The listing builds one solid part. Answer for the finished solid, in the listing's coordinates (mm). Give positions to 0.01 mm unless a question says otherwise; leave off trailing zeros. Order: outer loops, then holes, each group sorted by start corner. A loop starts at its lowest first (then second) coordinate and runs counter-clockwise, first axis right, second up. Notation, with made-up numbers: (85.5, -25.5) - (118.5, -25.5) arc R22 cw to (118.5, -15.5) - close; hole circle Ø3 at (-9, 80.5). An arc over 180 degrees is marked (long way). Use CSV: the item, a comma, the result in double quotes.
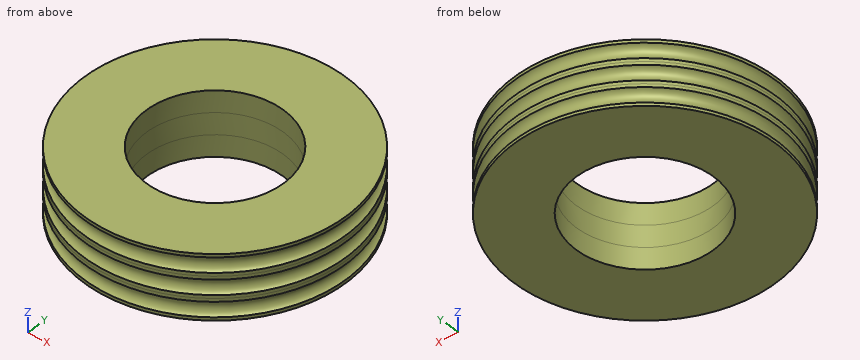
```python
from build123d import *


with BuildPart() as part:
    # Sketch2 → Revolve1 (revolve)
    with BuildSketch(Plane(origin=(0, 0, 0), x_dir=(0, 0, -1), z_dir=(1, 0, 0))):
        with BuildLine():
            Line((-0.34, 2.1), (-0.34, 4))
            Line((-0.34, 4), (-0.44, 4))
            ThreePointArc((-0.44, 4), (-0.67, 3.849201276), (-0.9, 4))
            Line((-0.9, 4), (-1, 4))
            Line((-1, 4), (-1, 2.1))
            Line((-1, 2.1), (-0.34, 2.1))
        make_face()
    revolve1 = revolve(axis=Axis((0, 0, 3.014677367), (0, 0, -1)))

    # Mirror2: Revolve1 across plane
    add(revolve1.mirror(Plane(origin=(0, 0, 0.34), x_dir=(1, 0, 0), z_dir=(0, 0, -1))))

    # Mirror3: Revolve1 across plane
    add(revolve1.mirror(Plane.XY.offset(1)))


solid = part.part
```
Item 1: The part is cut by section C-C (z = -0.1). Give the vertices of the cut face in (x, y), and give its area (3 significant figures).
Taken from the geometry:
outline,"circle Ø7.75 at (0, 0); hole circle Ø4.2 at (0, 0)"
area,"33.3 mm^2"
Item 2: Find the intervals of material crossed by line 1 along X through (y, z) = (0, -0.1); line 2 along Y through (x, z) = (0.75, 1.4); line 3 along X through (y, z) = (-1, 0.2), in increasing order.
Taken from the geometry:
line 1,"-3.87 to -2.1, 2.1 to 3.87"
line 2,"-3.79 to -1.96, 1.96 to 3.79"
line 3,"-3.81 to -1.85, 1.85 to 3.81"
Item 3: The part is cut by section A-A (y = 0). Give the vertices of the cut face in (x, z).
Taken from the geometry:
outline,"(-4, -0.32) - (-2.1, -0.32) - (-2.1, 1.66) - (-4, 1.66) - (-4, 1.56) arc R0.25 cw to (-4, 1.1) - (-4, 0.9) arc R0.25 cw to (-4, 0.44) - (-4, 0.24) arc R0.25 cw to (-4, -0.22) - close; (2.1, -0.32) - (4, -0.32) - (4, -0.22) arc R0.25 cw to (4, 0.24) - (4, 0.44) arc R0.25 cw to (4, 0.9) - (4, 1.1) arc R0.25 cw to (4, 1.56) - (4, 1.66) - (2.1, 1.66) - close"
